Autodesk Inventor part; units mm, degrees
ref_plane "YZ Plane" through (0, 0, 0) normal (1, 0, 0) x (0, 1, 0)
ref_plane "XZ Plane" through (0, 0, 0) normal (0, 1, 0) x (-1, 0, 0)
ref_plane "XY Plane" through (0, 0, 0) normal (0, 0, 1) x (1, 0, 0)
sketch "Sketch1" plane through (0, 0, 0) normal (0, 0, 1) x (1, 0, 0)
  line L0 (-30, 0) -> (30, 0)
  line L1 (30, 0) -> (30, 20)
  line L2 (-30, 20) -> (-30, 0)
  line L3 (60, 40) -> (60, 110)
  line L4 (60, 110) -> (-60, 110)
  line L5 (-60, 110) -> (-60, 40)
  line L6 (-60, 40) -> (-30, 20)
  line L7 (30, 20) -> (60, 40)
  point P0 (0, 0)
  dimension "d0" = 60
  dimension "d1" = 20
  dimension "d2" = 120
  dimension "d3" = 70
extrude "Extrusion1" add sketch "Sketch1" along normal blind 2
sketch "Sketch2" plane through (-30, 0, 0) normal (0, -1, 0) x (1, 0, 0)
  line L0 (60, 0) -> (60, 2)
  line L1 (60, 0) -> (0, 0)
  line L2 (0, 0) -> (0, -30)
  line L3 (0, -30) -> (60, -30)
  line L4 (60, -30) -> (60, 0)
  point P0 (30, 0)
  dimension "d6" = 60
  dimension "d7" = 30
extrude "Extrusion2" add sketch "Sketch2" against normal blind 2
sketch "Sketch3" plane through (0, 0, 2) normal (0, 0, 1) x (1, 0, 0)
  line L0 (-37, 90) -> (-29.0967, 76.3111)
  line L1 (-37, 90) -> (-21.1935, 90) construction
  line L2 (-30.5967, 76.3111) -> (-32.0967, 76.3111)
  line L3 (-32.0967, 76.3111) -> (-39.25, 88.701)
  line L4 (-39.25, 88.701) -> (-40, 90)
  line L5 (-40, 90) -> (-37, 90)
  line L6 (-29.0967, 76.3111) -> (-21.1935, 90)
  line L7 (-21.1935, 90) -> (-18.1935, 90)
  line L8 (-18.1935, 90) -> (-26.0967, 76.3111)
  line L9 (-26.0967, 76.3111) -> (-27.5967, 76.3111)
  line L10 (-30.5967, 76.3111) -> (-30.5967, 66.3111)
  line L11 (-30.5967, 66.3111) -> (-27.5967, 66.3111)
  line L12 (-27.5967, 66.3111) -> (-27.5967, 76.3111)
  line L13 (-14.1935, 90) -> (-14.1935, 66.3111)
  line L14 (-14.1935, 90) -> (-4.1935, 90)
  line L15 (-4.1935, 90) -> (-4.1935, 79.933)
  line L16 (-4.1935, 79.933) -> (-2.1935, 79.933)
  line L17 (-2.1935, 79.933) -> (-2.1935, 66.3111)
  line L18 (-2.1935, 66.3111) -> (-14.1935, 66.3111)
  line L19 (-10.757, 87) -> (-10.757, 82.506)
  line L20 (-10.757, 82.506) -> (-6.2868, 82.506)
  line L21 (-6.2868, 82.506) -> (-6.2868, 87)
  line L22 (-6.2868, 87) -> (-10.757, 87)
  line L23 (-10.757, 76.3111) -> (-10.757, 68.4995)
  line L24 (-10.757, 68.4995) -> (-3.7569, 68.4995)
  line L25 (-3.7569, 68.4995) -> (-3.7569, 76.3111)
  line L26 (-3.7569, 76.3111) -> (-10.757, 76.3111)
  line L27 (1.8065, 65.8916) -> (1.8065, 90)
  line L28 (1.8065, 90) -> (11.8065, 90)
  line L29 (11.8065, 90) -> (11.8065, 87)
  line L30 (11.8065, 87) -> (4.8065, 87)
  line L31 (4.8065, 87) -> (4.8065, 82)
  line L32 (4.8065, 82) -> (11.8065, 82)
  line L33 (11.8065, 82) -> (11.8065, 79)
  line L34 (11.8065, 79) -> (4.8065, 79)
  line L35 (4.8065, 79) -> (4.8065, 65.8916)
  line L36 (4.8065, 65.8916) -> (1.8065, 65.8916)
  line L37 (15.8065, 90) -> (15.8065, 64.9111)
  line L38 (15.8065, 64.9111) -> (30.8065, 64.9111)
  line L39 (30.8065, 64.9111) -> (30.8065, 67.9111)
  line L40 (30.8065, 67.9111) -> (18.8065, 67.9111)
  line L41 (18.8065, 67.9111) -> (18.8065, 90)
  line L42 (18.8065, 90) -> (15.8065, 90)
  point P0 (0, 0)
  dimension "d10" = 60
  dimension "d12" = 3
  dimension "d13" = 60
  dimension "d14" = 10
  dimension "d15" = 10
  dimension "d16" = 2
  dimension "d17" = 10
  dimension "d19" = 3
  dimension "d20" = 7
  dimension "d21" = 5
  dimension "d22" = 3
  dimension "d23" = 15
  dimension "d25" = 3
  dimension "d26" = 12
  dimension "d27" = 4
  dimension "d28" = 4
  dimension "d29" = 4
extrude "Extrusion3" cut sketch "Sketch3" against normal blind 2
sketch "Sketch6" plane through (0, 0, 2) normal (0, 0, 1) x (1, 0, 0)
  line L0 (-14.1935, 66.3111) -> (-2.1935, 66.3111)
  line L1 (-3.7569, 68.4995) -> (-5.7569, 68.4995)
  line L2 (-5.7569, 68.4995) -> (-5.7569, 66.3111)
  line L3 (-5.7569, 66.3111) -> (-3.7569, 66.3111)
  line L4 (-3.7569, 66.3111) -> (-3.7569, 68.4995)
  line L5 (-14.1935, 90) -> (-14.1935, 66.3111)
  line L6 (-10.757, 87) -> (-14.1935, 87)
  line L7 (-14.1935, 87) -> (-14.1935, 85)
  line L8 (-14.1935, 85) -> (-10.757, 85)
  line L9 (-10.757, 85) -> (-10.757, 87)
  point P0 (0, 0)
  dimension "d32" = 2
  dimension "d33" = 2
extrude "Extrusion4" add sketch "Sketch6" against normal blind 2
sketch "Sketch8" plane through (-60, 110, 0) normal (0, 1, 0) x (1, 0, 0)
  line L0 (45, 0) -> (75, 0)
  line L1 (75, 0) -> (75, 30)
  line L2 (75, 30) -> (45, 30)
  line L3 (45, 30) -> (45, 0)
  point P0 (60, 0)
  dimension "d36" = 30
  dimension "d37" = 30
extrude "Extrusion5" add sketch "Sketch8" against normal blind 2
sketch "Sketch9" plane through (-60, 40, 0) normal (-1, 0, 0) x (0, 0, 1)
  line L0 (0, 0) -> (0, 70)
  line L1 (0, 59.5) -> (-20, 59.5)
  line L2 (-20, 59.5) -> (-20, 50)
  line L3 (-20, 50) -> (0, 50)
  line L4 (0, 50) -> (0, 59.5)
  line L5 (0, 0) -> (2, 0)
  point P0 (0, -40)
  dimension "d40" = 20
  dimension "d41" = 9.5
  dimension "d56" = 50
extrude "Extrusion6" add sketch "Sketch9" against normal blind 2
sketch "Sketch10" plane through (-60, 40, 2) normal (-1, 0, 0) x (0, 0, 1)
  circle A0 centre (-16.7422, 57) radius 2.5
  line L0 (-2, 59.5) -> (-22, 59.5)
  line L1 (-22, 59.5) -> (-22, 50)
  circle A1 centre (-7.2426, 57) radius 2.5
  point P0 (-2, -40)
  dimension "d44" = 5
  dimension "d45" = 2.5
  dimension "d46" = 5.2578
  dimension "d47" = 5
  dimension "d48" = 2.5
  dimension "d49" = 9.4996
extrude "Extrusion7" cut sketch "Sketch10" against normal blind 2
sketch "Sketch12" plane through (60, 40, 0) normal (1, 0, 0) x (0, 0, -1)
  line L0 (5.2426, 59.5) -> (0, 59.5)
  line L1 (20, 50) -> (20, 59.5)
  line L2 (0, 59.5) -> (20, 59.5)
  line L3 (20, 59.5) -> (20, 50)
  line L4 (20, 50) -> (0, 50)
  line L5 (0, 50) -> (0, 59.5)
  point P0 (0, -40)
extrude "Extrusion8" add sketch "Sketch12" against normal blind 2
sketch "Sketch13" plane through (60, 40, 2) normal (1, 0, 0) x (0, 0, -1)
  circle A0 centre (7.2426, 57) radius 2.5
  circle A1 centre (7.2426, 57) radius 2.5
  circle A2 centre (16.7422, 57) radius 2.5
  circle A3 centre (16.7422, 57) radius 2.5
  point P0 (2, -40)
  point P1 (7.2426, 59.5)
  point P2 (16.7422, 59.5)
extrude "Extrusion9" cut sketch "Sketch13" against normal blind 2
properties part number "Body Front"
The model under review builds one solid part; all positions refer to its coordinate system, in mm. A direction names the side the tool comes from. Round coordinates to 2 decimals unless told otherwise and drop trailing zeros. Order: outer loops, then holes, each group sorted by start corner. A loop starts at its lowest first (then second) coordinate and runs counter-clockwise, first axis right, second up. Notation, with made-up numbers: (18, 59) - (63, 59) arc R19 ccw to (63, 82) - close; hole circle Ø5 at (29.5, 41). An arc over 180 degrees is marked (long way). Use one line per item in the form item = value.
Q1. Add section B-B on y = 71. Give the boundary of the cut face in (x, z), then the cut area to 3 significant figures.
Response values:
outline = (-60, 0) - (-30.6, 0) - (-30.6, 2) - (-60, 2) - close; (-27.6, 0) - (-14.19, 0) - (-14.19, 2) - (-27.6, 2) - close; (-10.76, 0) - (-3.76, 0) - (-3.76, 2) - (-10.76, 2) - close; (-2.19, 0) - (1.81, 0) - (1.81, 2) - (-2.19, 2) - close; (4.81, 0) - (15.81, 0) - (15.81, 2) - (4.81, 2) - close; (18.81, 0) - (60, 0) - (60, 2) - (18.81, 2) - close
area = 212 mm^2
Q2. Mouldability with a two-part tool opening along Y and no side actions: class faces 1 (the flat face through (58, 94, -10)), 2 (the flat face through (0, 110, -12)), 3 (the flat face through (0, 2, -15)), 4 (the flat face through (0, 0, -14)) as pulls with the +Y half, pulls with the -Y half, needs draft (parallel to the pull), parting line crosses it, or undercut.
Response values:
face_1 = needs draft
face_2 = pulls with the +Y half
face_3 = undercut
face_4 = pulls with the -Y half
Q3. Add section C-C on x = 45. Give the boundary of the cut face in (y, z), then the cut area to 3 significant figures.
Response values:
outline = (30, 0) - (110, 0) - (110, 2) - (30, 2) - close
area = 160 mm^2
Q4. To check wall thickness, follow line 1 (Z direction, x = -58.55, y = 97); line 2 (Y direction, x = -10.5, z = 1.5); line 3 (Y direction, x = -8, z = -22.5). State the ranges of each line that lie inside material, in increasing order.
Response values:
line_1 = -20 to -17.24, -12.24 to -7.74, -2.74 to 2
line_2 = 0 to 66.31, 68.5 to 76.31, 82.51 to 87, 90 to 110
line_3 = 0 to 2, 108 to 110
Q5. Add section D-D on y = 24.5. Give the boundary of the cut face in (x, z), then the cut area to 3 significant figures.
Response values:
outline = (-36.75, 0) - (36.75, 0) - (36.75, 2) - (-36.75, 2) - close
area = 147 mm^2
Q6. Add section A-A on z = -10. Give the boundary of the cut face in (x, y).
Response values:
outline = (-60, 90) - (-58, 90) - (-58, 99.5) - (-60, 99.5) - close; (-30, 0) - (30, 0) - (30, 2) - (-30, 2) - close; (-15, 108) - (15, 108) - (15, 110) - (-15, 110) - close; (58, 90) - (60, 90) - (60, 99.5) - (58, 99.5) - close
Q7. Clearance check with flat-ended pins moving along their axes: P1, Ø1, axis at x = -59.5, z = -3.5, coming from the +Y side; P2, Ø5, axis at y = 27, z = -1.5, coming from the +X side; P3, Ø2, axis at x = -59, z = -9, coming from the -Y side. State where each tip first meets the part, or that it passes through.
Response values:
P1 = 99.5
P2 = 43.5
P3 = 90
Q8. Tool access review of faces 5 (the flat face through (30, 1.8, -9.3)), 6 (the flat face through (-58, 94, -10)), 7 (the flat face through (0, 108, -15)), 8 (the flat face through (-30, 1, -8)), 9 (the flat face through (-33.104, 83.251, 1.014)): name each direction out of +Z, -Z, +X, -X, +Y, -Y from which nothing blocks a thin tool from reaching the whole face with its end or side.
Response values:
face_5 = +Z, -Z, +X, -Y
face_6 = -Z, +Y, -Y
face_7 = -Z, +X, -X
face_8 = +Z, -Z, -X, -Y
face_9 = +Z, -Z
